Input: part model. Units: mm. Frame: model coordinates. Face numbers are marked on the shaded views. A direction names the side the tool comes from. Give positions to 0.01 mm unless a question says otherwise; leave off trailing zeros. Loops run counter-clockwise (first coordinate to the right, second up) from the corner with the lowest first, then second, coordinate; pieces in that order, holes last. Notation, with made-up numbers: M -34,-37.75 L 8,-37.75 A23 ccw 8,1.25 Z; hole C 63.25,20 d8. An arc over 180 degrees is marked long. Return JSON: item names as keys, results as strings. Group by question number.
```python
from build123d import *

# Parameters (mm, degrees)
F0_R         = 4.5
F0_R_2       = 2.05
F1_DEPTH     = 12
F2_SIZE      = 0.3
F3_SIZE      = 0.5
F4_SIZE      = 0.5
F5_SIZE      = 0.3
F6_W         = 0.7801173814
F6_H         = 8
F8_S5_R      = 4.5
F8_T6_DEPTH  = 8
F8_S11_R     = 4.5
F8_T12_DEPTH = 8


# Not quite as in the source:
# - a fillet or chamfer that OpenCascade refuses, or shapes differently, is made with other operations: its cross-section is extruded or revolved along the edge and cut away or added


with BuildPart() as f1:
    # F0 (on Front) → F1 (new body)
    with BuildSketch(Plane.XZ):
        Circle(F0_R)
        Circle(F0_R_2, mode=Mode.SUBTRACT)
    extrude(amount=F1_DEPTH)

    # F2
    f2_edges = [f1.edges().sort_by_distance(p)[0] for p in [
        (-4.5, -12, 0),
    ]]
    chamfer(f2_edges, length=F2_SIZE)

    # F3
    f3_edges = [f1.edges().sort_by_distance(p)[0] for p in [
        (-2.05, -12, 0),
    ]]
    chamfer(f3_edges, length=F3_SIZE)

    # F4
    f4_edges = [f1.edges().sort_by_distance(p)[0] for p in [
        (-2.05, 0, 0),
    ]]
    chamfer(f4_edges, length=F4_SIZE)

    # F5
    f5_edges = [f1.edges().sort_by_distance(p)[0] for p in [
        (-4.5, 0, 0),
    ]]
    chamfer(f5_edges, length=F5_SIZE)

    # F6 (on Top) → F7 (revolve, cut)
    with BuildSketch(Plane.XY):
        with Locations((-4.1400586907, -6)):
            Rectangle(F6_W, F6_H)
    revolve(axis=Axis((0, 2.6414038148, 0), (0, 1, 0)), mode=Mode.SUBTRACT)

    # F8: chamfer of 1 on 3 edges, made by hand


with BuildPart() as f8_tool2:
    # F8_s3 → F8_t4 (revolve)
    with BuildSketch(Plane.XY):
        Polygon((-3.75, -9), (-4.75, -10), (-3.75, -10), align=None)
    revolve(axis=Axis((0, -10, 0), (0, 1, 0)))

    # F8_s5 → F8_t6 (intersect, symmetric)
    with BuildSketch(Plane.XZ.offset(9.5)):
        Circle(F8_S5_R)
    extrude(amount=F8_T6_DEPTH, both=True, mode=Mode.INTERSECT)


with BuildPart() as f1_1:
    add(f1.part)

    # F8_t1: union F8_tool2
    add(f8_tool2.part)


with BuildPart() as f8_tool8:
    # F8_s9 → F8_t10 (revolve)
    with BuildSketch(Plane.XY):
        Polygon((-4.75, -2), (-3.75, -3), (-3.75, -2), align=None)
    revolve(axis=Axis((0, -2, 0), (0, 1, 0)))

    # F8_s11 → F8_t12 (intersect, symmetric)
    with BuildSketch(Plane.XZ.offset(2.5)):
        Circle(F8_S11_R)
    extrude(amount=F8_T12_DEPTH, both=True, mode=Mode.INTERSECT)


with BuildPart() as f1_2:
    add(f1_1.part)

    # F8_t7: union F8_tool8
    add(f8_tool8.part)


solid = f1_2.part
```
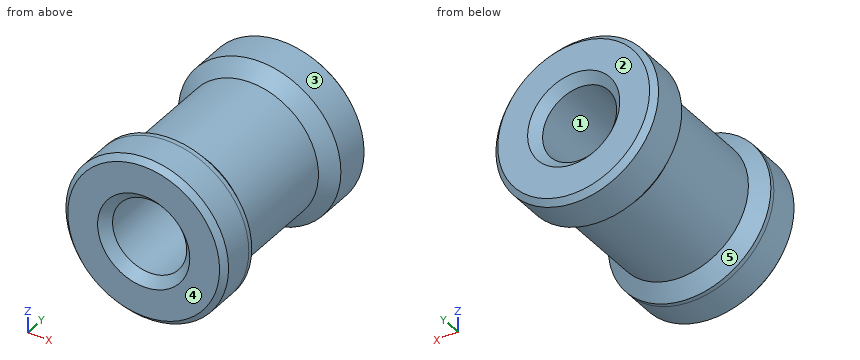
Item 1: Section D-D, the plane y = -0.75. Return loops of the section in (x, z), then the cut area to 3 significant figures.
Item 2: Section B-B, the plane z = 0. Return loops of the section in (x, y).
Item 3: Pull-direction query (Z, two-part tool) for the marked faces 1, 2 and 3; classes: pulls with the +Z half, pulls with the -Z half, needs draft (parallel to the pull), parting line crosses it, or undercut.
Item 4: Section A-A, the plane x = 0. Return loops of the section in (y, z).
Item 5: Section C-C, the plane y = -8. Return loops of the section in (x, z), then the cut area to 3 significant figures.
Item 6: First-contact query: pin 1 Ø2 at (x, z) = (-0.5, -2) entering from +Y; pin 2 Ø1 at (x, y) = (2.5, -5) entering from -Z; pin 3 Ø1 at (y, z) = (-10, 3) entering from -X. Flat tips, straight axial feed; report the tip coordinate or a pass-through.
Item 7: Reachability of the marked faces 4 and 5 from +Z, -Z, +X, -X, +Y, -Y: full face, straight path, thin tool, end or side. Return the list, or none.
Item 8: Material intervals for line 1 (X direction, y = -2.75, z = -1.25); line 2 (Z direction, x = 0, y = -2.75); line 3 (X direction, y = -7, z = 0.75), sorted ascending. Write a range as from..to.
Answer below:
{
 "1": {"outline": "C 0,0 d9; hole C 0,0 d4.1", "area": "50.4 mm^2"},
 "2": {"outline": "M -4.5,-11.7 L -4.2,-12 L -2.55,-12 L -2.05,-11.5 L -2.05,-0.5 L -2.55,0 L -4.2,0 L -4.5,-0.3 L -4.5,-2.25 L -3.75,-3 L -3.75,-9 L -4.5,-9.75 Z; M 2.05,-11.5 L 2.55,-12 L 4.2,-12 L 4.5,-11.7 L 4.5,-9.75 L 3.75,-9 L 3.75,-3 L 4.5,-2.25 L 4.5,-0.3 L 4.2,0 L 2.55,0 L 2.05,-0.5 Z"},
 "3": {"face 1": "undercut", "face 2": "needs draft", "face 3": "parting line crosses it"},
 "4": {"outline": "M -12,-4.2 L -11.7,-4.5 L -9.75,-4.5 L -9,-3.75 L -3,-3.75 L -2.25,-4.5 L -0.3,-4.5 L 0,-4.2 L 0,-2.55 L -0.5,-2.05 L -11.5,-2.05 L -12,-2.55 Z; M -12,2.55 L -11.5,2.05 L -0.5,2.05 L 0,2.55 L 0,4.2 L -0.3,4.5 L -2.25,4.5 L -3,3.75 L -9,3.75 L -9.75,4.5 L -11.7,4.5 L -12,4.2 Z"},
 "5": {"outline": "C 0,0 d7.5; hole C 0,0 d4.1", "area": "31.0 mm^2"},
 "6": {"pin 1": "y = 0", "pin 2": "z = -3.17", "pin 3": "x = -3.74"},
 "7": {"face 4": "+Z, -Z, +X, -X, -Y", "face 5": "none"},
 "8": {"line 1": "-3.8..-1.62, 1.62..3.8", "line 2": "-4..-2.05, 2.05..4", "line 3": "-3.67..-1.91, 1.91..3.67"}
}
